Source: CAD feature listing. Evaluate the final solid. Frame: model axes, mm. A direction names the side the tool comes from. Round coordinates to 2 decimals unless told otherwise and drop trailing zeros. Order: outer loops, then holes, each group sorted by start corner. A loop starts at its lowest first (then second) coordinate and runs counter-clockwise, first axis right, second up. Notation, with made-up numbers: (8.25, -17.75) - (42.25, -17.75) arc R36 cw to (42.25, 18.25) - close; hole circle Ø11 at (70, 5.5). An arc over 180 degrees is marked (long way). Return JSON: item names as keys, results as strings. Group by question number.
1) Section B-B, the plane y = 13.5. Return loops of the section in (x, z).
2) Section A-A, the plane x = 86. Return loops of the section in (y, z).
3) Ray query, line 1 (Y direction, x = 32.5, z = 26); line 2 (Y direction, x = 82.5, z = 3); line 3 (X direction, y = 24, z = 48). Return the intervals inside material, ascending. Write a range as from..to.
4) Access query for faces 4 (the flat face through (95.211, 26, 7)), 5 (the flat face through (92.211, 26, 42)), 6 (the flat face through (80.524, 0.822, 24.86)), 7 (the flat face through (76, 2, 55)). Directions: +Z, -Z, +X, -X, +Y, -Y. A direction counts if a zero-diameter tool reaches every point of the face in a straight line with its end or side. Return the directions, or none.
5) Contact query for flat-ended pins moving along their axis: P1, Ø4, axis at y = 13, z = 46, coming from the -X side; P2, Ø2, axis at x = 61, z = 11.5, coming from the +Y side; P3, Ø11.5, axis at x = 90.5, y = 20.5, coming from the -Z side. Output: stop coordinate, or through.
6) Section C-C, the plane z = 4. Return loops of the section in (x, y).
7) Mould query, pull axis Z, two halves, no side actions, for faces 1 (the flat face through (91, 22, 15)), 2 (the flat face through (40, 2, -10)), 3 (the flat face through (86.19, 14.06, 42.4)). Classes: pulls with the +Z half, pulls with the -Z half, needs draft (parallel to the pull), parting line crosses it, or undercut.
8) Section D-D, the plane z = 53. Return loops of the section in (x, y), plus the area to 3 significant figures.
```python
from build123d import *

# Parameters (mm, degrees)
SKETCH1_R               = 5
BOSS_EXTRUDE1_DEPTH     = 50
SKETCH2_R               = 2
CUT_EXTRUDE1_DEPTH      = 51
SKETCH7_W               = 20
SKETCH7_H               = 39.987182744
CUT_EXTRUDE3_DEPTH      = 10
CUT_EXTRUDE3_DEPTH_BACK = 10
BOSS_EXTRUDE2_REACH     = 52
CUT_EXTRUDE4_REACH      = 100.711
SKETCH9_W               = 20
SKETCH9_H               = 10.896319728
CUT_EXTRUDE6_REACH      = 52
SKETCH11_W              = 5
SKETCH11_H              = 3
SKETCH12_W              = 71
SKETCH12_H              = 70
BOSS_EXTRUDE3_DEPTH     = 3


with BuildPart() as part:
    # Sketch1 → Boss-Extrude1 (new body)
    with BuildSketch(Plane.XY):
        with Locations((93.71075113, 32.460861794)):
            Circle(SKETCH1_R)
        Polygon((0, 3), (0, 0), (81.758772051, 0), (95.21075113, 24.032587983), (95.21075113, 29.815076366), (92.21075113, 29.815076366), (92.21075113, 24.815076366), (80, 3), align=None)
    extrude(amount=BOSS_EXTRUDE1_DEPTH)

    # Sketch2 → Cut-Extrude1 (cut, through all)
    with BuildSketch(Plane.XY):
        with Locations((93.71075113, 32.460861794)):
            Circle(SKETCH2_R)
    extrude(amount=CUT_EXTRUDE1_DEPTH, mode=Mode.SUBTRACT)

    # Sketch7 → Cut-Extrude3 (cut, two sides)
    with BuildSketch(Plane(origin=(62.254079791, -34.846042362, 0), x_dir=(0, 0, -1), z_dir=(0.872603055, -0.488430045, 0))) as cut_extrude3_sk:
        with Locations((-25, 59.927032101)):
            Rectangle(SKETCH7_W, SKETCH7_H)
    extrude(amount=CUT_EXTRUDE3_DEPTH, mode=Mode.SUBTRACT)
    extrude(cut_extrude3_sk.sketch, amount=-CUT_EXTRUDE3_DEPTH_BACK, mode=Mode.SUBTRACT)

    # Sketch8 → Boss-Extrude2 (add, up to next)
    with BuildSketch(Plane.XY, mode=Mode.PRIVATE) as boss_extrude2_sk1:
        Polygon((66.951015515, 3), (66.951015515, 0), (81.758772051, 0), (79.25400484, 1.667244856), (80, 3), align=None)
    boss_extrude2_tool1 = extrude(boss_extrude2_sk1.sketch, amount=BOSS_EXTRUDE2_REACH, mode=Mode.PRIVATE) - part.part
    add(boss_extrude2_tool1.solids().sort_by_distance((73.552437, 1.463367, 0))[0])

    # Sketch9 → Cut-Extrude4 (cut, up to next)
    with BuildSketch(Plane(origin=(0, 0, 0), x_dir=(0, 0, -1), z_dir=(1, 0, 0)), mode=Mode.PRIVATE) as cut_extrude4_sk1:
        with Locations((-25, 32.01270193)):
            Rectangle(SKETCH9_W, SKETCH9_H)
    cut_extrude4_tool1 = extrude(cut_extrude4_sk1.sketch, amount=CUT_EXTRUDE4_REACH, mode=Mode.PRIVATE) & part.part
    add(cut_extrude4_tool1.solids().sort_by_distance((0, 32.012702, 25))[0], mode=Mode.SUBTRACT)

    # Sketch11 → Cut-Extrude6 (cut, up to next)
    with BuildSketch(Plane.XY.offset(50), mode=Mode.PRIVATE) as cut_extrude6_sk1:
        with Locations((2.5, 1.5)):
            Rectangle(SKETCH11_W, SKETCH11_H)
    cut_extrude6_tool1 = extrude(cut_extrude6_sk1.sketch, amount=-CUT_EXTRUDE6_REACH, mode=Mode.PRIVATE) & part.part
    add(cut_extrude6_tool1.solids().sort_by_distance((2.5, 1.5, 50))[0], mode=Mode.SUBTRACT)

    # Sketch12 → Boss-Extrude3 (add, through all)
    with BuildSketch(Plane(origin=(0, 3, 0), x_dir=(1, 0, 0), z_dir=(0, 1, 0))):
        with Locations((40.5, -25)):
            Rectangle(SKETCH12_W, SKETCH12_H)
    extrude(amount=-BOSS_EXTRUDE3_DEPTH)


solid = part.part
```
Geometry check:
{
 "1": {"outline": "(85.88, 0) - (89.32, 0) - (89.32, 15) - (85.88, 15) - close; (85.88, 35) - (89.32, 35) - (89.32, 50) - (85.88, 50) - close"},
 "2": {"outline": "(7.58, 0) - (13.72, 0) - (13.72, 15) - (7.58, 15) - close; (7.58, 35) - (13.72, 35) - (13.72, 50) - (7.58, 50) - close"},
 "3": {"line 1": "0..3", "line 2": "1.32..7.47", "line 3": "91.75..95.19"},
 "4": {"face 4": "+Z, -Z, +X, -Y", "face 5": "+Z, -Z, -X", "face 6": "+X", "face 7": "+Z, +X, +Y, -Y"},
 "5": {"P1": "x = 84.48", "P2": "y = 3", "P3": "z = 0"},
 "6": {"outline": "(5, 0) - (81.76, 0) - (95.21, 24.03) - (95.21, 27.69) arc R5 ccw (long way) to (92.21, 27.69) - (92.21, 24.82) - (80, 3) - (5, 3) - close; hole circle Ø4 at (93.71, 32.46)"},
 "7": {"face 1": "undercut", "face 2": "pulls with the -Z half", "face 3": "needs draft"},
 "8": {"outline": "(5, 0) - (76, 0) - (76, 3) - (5, 3) - close", "area": "213 mm2"}
}
